```python
from build123d import *

# Parameters (mm, degrees)
CROQUIS1_R                                           = 132.5
SALIENTE_EXTRUIR1_DEPTH                              = 5
CORTAR_EXTRUIR4_START                                = -5
CORTAR_EXTRUIR4_DEPTH                                = 5
AVELLANADO_PARA_TORNILLO_CON_CABEZA_PLAN_D           = 4.5
AVELLANADO_PARA_TORNILLO_CON_CABEZA_PLAN_CSINK_D     = 9.4
AVELLANADO_PARA_TORNILLO_CON_CABEZA_PLAN_CSINK_ANGLE = 90
AVELLANADO_PARA_TORNILLO_CON_CABEZA_2_D              = 6.6
AVELLANADO_PARA_TORNILLO_CON_CABEZA_2_CSINK_D        = 12.6
AVELLANADO_PARA_TORNILLO_CON_CABEZA_2_CSINK_ANGLE    = 90
AVELLANADO_PARA_TORNILLO_CON_CABEZA_3_D              = 4.8
AVELLANADO_PARA_TORNILLO_CON_CABEZA_3_CSINK_D        = 9.4
AVELLANADO_PARA_TORNILLO_CON_CABEZA_3_CSINK_ANGLE    = 90
CROQUIS32_W                                          = 85
CROQUIS32_H                                          = 35
SALIENTE_EXTRUIR6_DEPTH                              = 14.5
CORTAR_EXTRUIR8_REACH                                = 266.425
CROQUIS33_R                                          = 14.5
CORTAR_EXTRUIR9_START                                = -208
CROQUIS34_W                                          = 35
CROQUIS34_H                                          = 5.5
CORTAR_EXTRUIR9_DEPTH                                = 208
CHAFL_N2_SIZE                                        = 2
CROQUIS35_W                                          = 80
CROQUIS35_H                                          = 73
CROQUIS35_W_2                                        = 77
CROQUIS35_H_2                                        = 70
SALIENTE_EXTRUIR7_DEPTH                              = 25
SALIENTE_EXTRUIR8_START                              = 3
CROQUIS36_R                                          = 3.75
CROQUIS36_R_2                                        = 2.25
SALIENTE_EXTRUIR8_DEPTH                              = 3


with BuildPart() as part:
    # Croquis1 → Saliente-Extruir1 (new body)
    with BuildSketch(Plane(origin=(0, 0, 0), x_dir=(1, 0, 0), z_dir=(0, 1, 0))):
        with Locations(Location((0, 0, 0), (0, 0, 270))):
            Circle(CROQUIS1_R)
    extrude(amount=SALIENTE_EXTRUIR1_DEPTH)

    # Croquis6 → Cortar-Extruir4 (cut)
    with BuildSketch(Plane(origin=(0, 5, 0), x_dir=(1, 0, 0), z_dir=(0, 1, 0)).offset(CORTAR_EXTRUIR4_START)):
        with BuildLine():
            Line((-104, 46.693147249), (-104, -46.693147249))
            Line((-104, -46.693147249), (-124, -46.693147249))
            ThreePointArc((-124, -46.693147249), (-132.5, 0), (-124, 46.693147249))
            Line((-124, 46.693147249), (-104, 46.693147249))
        make_face()
        with BuildLine():
            Line((104, 46.693147249), (104, -46.693147249))
            Line((104, -46.693147249), (124, -46.693147249))
            ThreePointArc((124, -46.693147249), (132.5, 0), (124, 46.693147249))
            Line((124, 46.693147249), (104, 46.693147249))
        make_face()
    extrude(amount=CORTAR_EXTRUIR4_DEPTH, mode=Mode.SUBTRACT)

    # Avellanado para tornillo con cabeza plan (through all)
    with Locations(Plane(origin=(0, 0, 0), x_dir=(-1, 0, 0), z_dir=(0, -1, 0))):
        with Locations((70, 30), (12, 30), (70, 79), (12, 79)):
            CounterSinkHole(AVELLANADO_PARA_TORNILLO_CON_CABEZA_PLAN_D / 2, AVELLANADO_PARA_TORNILLO_CON_CABEZA_PLAN_CSINK_D / 2, counter_sink_angle=AVELLANADO_PARA_TORNILLO_CON_CABEZA_PLAN_CSINK_ANGLE)

    # Avellanado para tornillo con cabeza  2 (through all)
    with Locations(Plane(origin=(87, 0, 45), x_dir=(0, 0, -1), z_dir=(0, -1, 0))):
        with Locations((0, 0), (0, -173.856203002), (89.72135955, -173.856203002), (89.72135955, 0)):
            CounterSinkHole(AVELLANADO_PARA_TORNILLO_CON_CABEZA_2_D / 2, AVELLANADO_PARA_TORNILLO_CON_CABEZA_2_CSINK_D / 2, counter_sink_angle=AVELLANADO_PARA_TORNILLO_CON_CABEZA_2_CSINK_ANGLE)

    # Avellanado para tornillo con cabeza  3 (through all)
    with Locations(Plane(origin=(0, 5, 0), x_dir=(1, 0, 0), z_dir=(0, 1, 0))):
        with Locations((-20, -100), (20, -100), (-20, 100), (20, 100)):
            CounterSinkHole(AVELLANADO_PARA_TORNILLO_CON_CABEZA_3_D / 2, AVELLANADO_PARA_TORNILLO_CON_CABEZA_3_CSINK_D / 2, counter_sink_angle=AVELLANADO_PARA_TORNILLO_CON_CABEZA_3_CSINK_ANGLE)

    # Croquis32 → Saliente-Extruir6 (add)
    with BuildSketch(Plane(origin=(0, 5, 0), x_dir=(1, 0, 0), z_dir=(0, 1, 0))):
        with Locations((61.5, 0)):
            Rectangle(CROQUIS32_W, CROQUIS32_H)
        with Locations((-61.5, 0)):
            Rectangle(CROQUIS32_W, CROQUIS32_H)
    extrude(amount=SALIENTE_EXTRUIR6_DEPTH)

    # Cortar-Extruir8: up to this face of the body (flat: up to its plane)
    cortar_extruir8_end = Plane(part.part.faces().sort_by_distance((104, 7.577960985, 0))[0])
    # Croquis33 → Cortar-Extruir8 (cut, up to the picked face)
    with BuildSketch(Plane.ZY.offset(104), mode=Mode.PRIVATE) as cortar_extruir8_sk1:
        with Locations((0, 19.5)):
            Circle(CROQUIS33_R)
    cortar_extruir8_tool1 = split(extrude(cortar_extruir8_sk1.sketch, amount=-CORTAR_EXTRUIR8_REACH, mode=Mode.PRIVATE), bisect_by=cortar_extruir8_end, keep=Keep.BOTH, mode=Mode.PRIVATE)
    add(cortar_extruir8_tool1.solids().sort_by(Axis((-104, 19.5, 0), (1, 0, 0)))[0], mode=Mode.SUBTRACT)

    # Croquis34 → Cortar-Extruir9 (cut)
    with BuildSketch(Plane.ZY.offset(104).offset(CORTAR_EXTRUIR9_START)):
        with Locations((0, 16.75)):
            Rectangle(CROQUIS34_W, CROQUIS34_H)
    extrude(amount=CORTAR_EXTRUIR9_DEPTH, mode=Mode.SUBTRACT)

    # Chaflán2
    # the kernel refuses this chamfer: 2 mm, written as the material it adds along each edge
    with BuildSketch(Plane(origin=(104, 5, -17.5), x_dir=(0, 0, -1), z_dir=(-1, 0, 0)), Plane(origin=(19, 5, 17.5), x_dir=(0, 0, 1), z_dir=(1, 0, 0))) as chafl_n2_piece_1:
        Polygon((CHAFL_N2_SIZE, 0), (0, -CHAFL_N2_SIZE), (0, 0), align=None)
    extrude(amount=85)
    with BuildSketch(Plane(origin=(19, 5, -17.5), x_dir=(-1, 0, 0), z_dir=(0, 0, 1))) as chafl_n2_piece_2_section:
        Polygon((CHAFL_N2_SIZE, 0), (0, -CHAFL_N2_SIZE), (0, 0), align=None)
    chafl_n2_piece_2 = extrude(amount=17.5, mode=Mode.PRIVATE)
    chafl_n2_piece_2 = chafl_n2_piece_2 - Plane(origin=(19, 19.5, 0), x_dir=(0, 0, 1), z_dir=(-1, 0, 0)) * Cylinder(14.5, 43, mode=Mode.PRIVATE)
    add(chafl_n2_piece_2)
    with BuildSketch(Plane(origin=(-19, 5, 17.5), x_dir=(0, 0, 1), z_dir=(-1, 0, 0)), Plane(origin=(-104, 5, -17.5), x_dir=(0, 0, -1), z_dir=(1, 0, 0))) as chafl_n2_piece_3:
        Polygon((CHAFL_N2_SIZE, 0), (0, CHAFL_N2_SIZE), (0, 0), align=None)
    extrude(amount=85)
    with BuildSketch(Plane(origin=(-19, 5, 0), x_dir=(1, 0, 0), z_dir=(0, 0, 1))) as chafl_n2_piece_4_section:
        Polygon((CHAFL_N2_SIZE, 0), (0, CHAFL_N2_SIZE), (0, 0), align=None)
    chafl_n2_piece_4 = extrude(amount=17.5, mode=Mode.PRIVATE)
    chafl_n2_piece_4 = chafl_n2_piece_4 - Plane(origin=(-19, 19.5, 0), x_dir=(0, 0, 1), z_dir=(-1, 0, 0)) * Cylinder(14.5, 44, mode=Mode.PRIVATE)
    add(chafl_n2_piece_4)
    with BuildSketch(Plane(origin=(-19, 5, -17.5), x_dir=(1, 0, 0), z_dir=(0, 0, 1))) as chafl_n2_piece_5_section:
        Polygon((CHAFL_N2_SIZE, 0), (0, CHAFL_N2_SIZE), (0, 0), align=None)
    chafl_n2_piece_5 = extrude(amount=17.5, mode=Mode.PRIVATE)
    chafl_n2_piece_5 = chafl_n2_piece_5 - Plane(origin=(-19, 19.5, 0), x_dir=(0, 0, 1), z_dir=(-1, 0, 0)) * Cylinder(14.5, 43, mode=Mode.PRIVATE)
    add(chafl_n2_piece_5)
    with BuildSketch(Plane(origin=(19, 5, 0), x_dir=(-1, 0, 0), z_dir=(0, 0, 1))) as chafl_n2_piece_6_section:
        Polygon((CHAFL_N2_SIZE, 0), (0, -CHAFL_N2_SIZE), (0, 0), align=None)
    chafl_n2_piece_6 = extrude(amount=17.5, mode=Mode.PRIVATE)
    chafl_n2_piece_6 = chafl_n2_piece_6 - Plane(origin=(19, 19.5, 0), x_dir=(0, 0, 1), z_dir=(-1, 0, 0)) * Cylinder(14.5, 44, mode=Mode.PRIVATE)
    add(chafl_n2_piece_6)
    with BuildSketch(Plane(origin=(19, 5, -22.643365976), x_dir=(-1, 0, 0), z_dir=(0, 0, 1))) as chafl_n2_piece_7a_section:
        Polygon((CHAFL_N2_SIZE, 0), (0, -CHAFL_N2_SIZE), (0, 0), align=None)
    chafl_n2_piece_7a = extrude(amount=22.643365976, mode=Mode.PRIVATE)
    chafl_n2_piece_7a = split(chafl_n2_piece_7a, bisect_by=Plane(origin=(19, 5, -17.5), z_dir=(0, 0, -1)), keep=Keep.TOP, mode=Mode.PRIVATE)
    with BuildSketch(Plane(origin=(104, 5, -17.5), x_dir=(0, 0, -1), z_dir=(-1, 0, 0))) as chafl_n2_piece_7b_section:
        Polygon((CHAFL_N2_SIZE, 0), (0, -CHAFL_N2_SIZE), (0, 0), align=None)
    chafl_n2_piece_7b = extrude(amount=90.143365976, mode=Mode.PRIVATE)
    chafl_n2_piece_7b = split(chafl_n2_piece_7b, bisect_by=Plane(origin=(19, 5, -17.5), z_dir=(-1, 0, 0)), keep=Keep.TOP, mode=Mode.PRIVATE)
    chafl_n2_piece_7 = chafl_n2_piece_7a & chafl_n2_piece_7b
    add(chafl_n2_piece_7)
    with BuildSketch(Plane(origin=(13.856634024, 5, 17.5), x_dir=(0, 0, 1), z_dir=(1, 0, 0))) as chafl_n2_piece_8a_section:
        Polygon((CHAFL_N2_SIZE, 0), (0, -CHAFL_N2_SIZE), (0, 0), align=None)
    chafl_n2_piece_8a = extrude(amount=90.143365976, mode=Mode.PRIVATE)
    chafl_n2_piece_8a = split(chafl_n2_piece_8a, bisect_by=Plane(origin=(19, 5, 17.5), z_dir=(-1, 0, 0)), keep=Keep.TOP, mode=Mode.PRIVATE)
    with BuildSketch(Plane(origin=(19, 5, 0), x_dir=(-1, 0, 0), z_dir=(0, 0, 1))) as chafl_n2_piece_8b_section:
        Polygon((CHAFL_N2_SIZE, 0), (0, -CHAFL_N2_SIZE), (0, 0), align=None)
    chafl_n2_piece_8b = extrude(amount=22.643365976, mode=Mode.PRIVATE)
    chafl_n2_piece_8b = split(chafl_n2_piece_8b, bisect_by=Plane(origin=(19, 5, 17.5), z_dir=(0, 0, 1)), keep=Keep.TOP, mode=Mode.PRIVATE)
    chafl_n2_piece_8 = chafl_n2_piece_8a & chafl_n2_piece_8b
    add(chafl_n2_piece_8)
    with BuildSketch(Plane(origin=(-13.856634024, 5, 17.5), x_dir=(0, 0, 1), z_dir=(-1, 0, 0))) as chafl_n2_piece_9a_section:
        Polygon((CHAFL_N2_SIZE, 0), (0, CHAFL_N2_SIZE), (0, 0), align=None)
    chafl_n2_piece_9a = extrude(amount=90.143365976, mode=Mode.PRIVATE)
    chafl_n2_piece_9a = split(chafl_n2_piece_9a, bisect_by=Plane(origin=(-19, 5, 17.5), z_dir=(1, 0, 0)), keep=Keep.TOP, mode=Mode.PRIVATE)
    with BuildSketch(Plane(origin=(-19, 5, 0), x_dir=(1, 0, 0), z_dir=(0, 0, 1))) as chafl_n2_piece_9b_section:
        Polygon((CHAFL_N2_SIZE, 0), (0, CHAFL_N2_SIZE), (0, 0), align=None)
    chafl_n2_piece_9b = extrude(amount=22.643365976, mode=Mode.PRIVATE)
    chafl_n2_piece_9b = split(chafl_n2_piece_9b, bisect_by=Plane(origin=(-19, 5, 17.5), z_dir=(0, 0, 1)), keep=Keep.TOP, mode=Mode.PRIVATE)
    chafl_n2_piece_9 = chafl_n2_piece_9a & chafl_n2_piece_9b
    add(chafl_n2_piece_9)
    with BuildSketch(Plane(origin=(-104, 5, -17.5), x_dir=(0, 0, -1), z_dir=(1, 0, 0))) as chafl_n2_piece_10a_section:
        Polygon((CHAFL_N2_SIZE, 0), (0, CHAFL_N2_SIZE), (0, 0), align=None)
    chafl_n2_piece_10a = extrude(amount=90.143365976, mode=Mode.PRIVATE)
    chafl_n2_piece_10a = split(chafl_n2_piece_10a, bisect_by=Plane(origin=(-19, 5, -17.5), z_dir=(1, 0, 0)), keep=Keep.TOP, mode=Mode.PRIVATE)
    with BuildSketch(Plane(origin=(-19, 5, -22.643365976), x_dir=(1, 0, 0), z_dir=(0, 0, 1))) as chafl_n2_piece_10b_section:
        Polygon((CHAFL_N2_SIZE, 0), (0, CHAFL_N2_SIZE), (0, 0), align=None)
    chafl_n2_piece_10b = extrude(amount=22.643365976, mode=Mode.PRIVATE)
    chafl_n2_piece_10b = split(chafl_n2_piece_10b, bisect_by=Plane(origin=(-19, 5, -17.5), z_dir=(0, 0, -1)), keep=Keep.TOP, mode=Mode.PRIVATE)
    chafl_n2_piece_10 = chafl_n2_piece_10a & chafl_n2_piece_10b
    add(chafl_n2_piece_10)

    # Croquis35 → Saliente-Extruir7 (add)
    with BuildSketch(Plane(origin=(0, 5, 0), x_dir=(1, 0, 0), z_dir=(0, 1, 0))):
        with Locations((0, -57.5)):
            Rectangle(CROQUIS35_W, CROQUIS35_H)
        with Locations((0, -57.5)):
            Rectangle(CROQUIS35_W_2, CROQUIS35_H_2, mode=Mode.SUBTRACT)
    extrude(amount=SALIENTE_EXTRUIR7_DEPTH)

    # Croquis36 → Saliente-Extruir8 (add)
    # profile 1 of 4: a face of its own
    with BuildSketch(Plane(origin=(0, 5, 0), x_dir=(1, 0, 0), z_dir=(0, 1, 0)).offset(SALIENTE_EXTRUIR8_START)):
        with Locations(Location((-70, 79, 0), (0, 0, 270))):
            Circle(CROQUIS36_R)
        with Locations(Location((-70, 79, 0), (0, 0, 90))):
            Circle(CROQUIS36_R_2, mode=Mode.SUBTRACT)
    # profile 2 of 4: a face of its own
    with BuildSketch(Plane(origin=(0, 5, 0), x_dir=(1, 0, 0), z_dir=(0, 1, 0)).offset(SALIENTE_EXTRUIR8_START)):
        with Locations(Location((-12, 79, 0), (0, 0, 270))):
            Circle(CROQUIS36_R)
        with Locations(Location((-12, 79, 0), (0, 0, 90))):
            Circle(CROQUIS36_R_2, mode=Mode.SUBTRACT)
    # profile 3 of 4: a face of its own
    with BuildSketch(Plane(origin=(0, 5, 0), x_dir=(1, 0, 0), z_dir=(0, 1, 0)).offset(SALIENTE_EXTRUIR8_START)):
        with Locations(Location((-12, 30, 0), (0, 0, 270))):
            Circle(CROQUIS36_R)
        with Locations(Location((-12, 30, 0), (0, 0, 90))):
            Circle(CROQUIS36_R_2, mode=Mode.SUBTRACT)
    # profile 4 of 4: a face of its own
    with BuildSketch(Plane(origin=(0, 5, 0), x_dir=(1, 0, 0), z_dir=(0, 1, 0)).offset(SALIENTE_EXTRUIR8_START)):
        with Locations(Location((-70, 30, 0), (0, 0, 270))):
            Circle(CROQUIS36_R)
        with Locations(Location((-70, 30, 0), (0, 0, 90))):
            Circle(CROQUIS36_R_2, mode=Mode.SUBTRACT)
    extrude(amount=-SALIENTE_EXTRUIR8_DEPTH)


solid = part.part
```
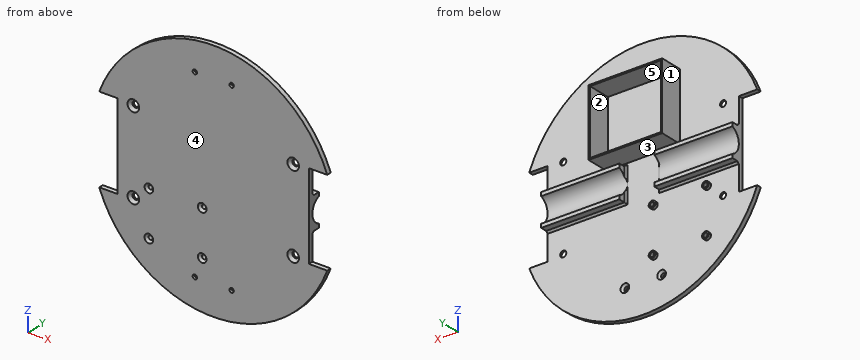
Model file for the job. Use its own axes, mm. Face numbers are marked on the shaded views. A direction names the side the tool comes from. Round coordinates to 2 decimals unless told otherwise and drop trailing zeros. Loops run counter-clockwise (first coordinate to the right, second up) from the corner with the lowest first, then second, coordinate; pieces in that order, holes last. Notation, with made-up numbers: M 46.5,30.5 L 96.5,30.5 A15 cw 96.5,38.5 Z; hole C 58,64 d2. An arc over 180 degrees is marked long. Put each result on its own line as item: value. Start each with the question number.
Item 1: Mould opens along Z. For the marked faces 1 and 2 say: released by +Z, released by -Z, zero draft, split by the parting line, or undercut.
Item 2: Drill centre lines: line 1 along X through (y, z) = (3.75, -30); line 2 along X through (y, z) = (4.1, 45); line 3 along Z through (x, y) = (20, 1.35). Where is each one in solid material? Low to high.
Item 3: Drop flat-ended pins along their axis: P1, Ø5.5, axis at y = 10, z = -13, coming from the +X side; P2, Ø12, axis at x = 30, z = -11, coming from the -Y side; P3, Ø8, axis at x = -71.5, z = -31, coming from the +Y side; P4, Ø8.5, axis at x = -86.86, z = -44.72, coming from the -Y side. Give the stop position or say it passes through.
Item 4: Cut at B-B (x = 87). List the corners of the cut face in (y, z), then the cut area to 3 significant figures.
Item 5: Cut at A-A (z = 27.5). List the corners of the cut face in (x, y), then the cut area to 4 significant figures.
Item 6: Cut at C-C (x = -4). List the corners of the cut face in (y, z), then the cut area to 3 significant figures.
Item 7: 3-axis set-ups, long thin cutter, end or side, ignore diameter. For the marked faces 3, 4 and 5: which of +Z, -Z, +X, -X, +Y, -Y reach the whole face in a straight line?
Item 8: Cut at D-D (z = -65.5). List the corners of the cut face in (x, y), then the cut area to 3 significant figures.
Answer block:
1. face 1: zero draft
1. face 2: undercut
2. line 1: -104 to -72.25, -67.75 to -14.25, -9.75 to 104
2. line 2: -104 to -90.16, -83.56 to 83.7, 90.3 to 104
2. line 3: -130.98 to -102.4, -97.6 to 97.6, 102.4 to 130.98
3. P1: x = 104
3. P2: y = 0
3. P3: y = 8
3. P4: y = 2.05
4. outline: M 0,-99.94 L 5,-99.94 L 5,-48.02 L 3,-48.02 L 0,-51.02 Z; M 0,-38.42 L 3,-41.42 L 5,-41.42 L 5,-19.5 L 7,-17.5 L 14,-17.5 L 14,-13.42 A14.5 cw 14,13.42 L 14,17.5 L 7,17.5 L 5,19.5 L 5,41.7 L 3,41.7 L 0,38.7 Z; M 0,51.3 L 3,48.3 L 5,48.3 L 5,99.94 L 0,99.94 Z
4. area: 1,060 mm2
5. outline: M -104,0 L 104,0 L 104,5 L 40,5 L 40,30 L 38.5,30 L 38.5,5 L -38.5,5 L -38.5,30 L -40,30 L -40,5 L -104,5 Z
5. area: 1,115 mm2
6. outline: M 0,-132.44 L 5,-132.44 L 5,21 L 30,21 L 30,22.5 L 5,22.5 L 5,92.5 L 30,92.5 L 30,94 L 5,94 L 5,132.44 L 0,132.44 Z
6. area: 1,400 mm2
7. face 3: +X, -X, +Y
7. face 4: +Z, -Z, +X, -X, -Y
7. face 5: +Y
8. outline: M -115.18,0 L 115.18,0 L 115.18,5 L -115.18,5 Z
8. area: 1,150 mm2
